Here's how the part is built. I have some questions about the finished solid (model axes, mm). A direction names the side the tool comes from. Round coordinates to 2 decimals unless told otherwise and drop trailing zeros. Order: outer loops, then holes, each group sorted by start corner. A loop starts at its lowest first (then second) coordinate and runs counter-clockwise, first axis right, second up.
```python
from build123d import *

# Parameters (mm, degrees)
F1_W     = 30
F1_H     = 32.3
F2_DEPTH = 7
F0_W     = 12.5
F0_H     = 22.6
F3_DEPTH = 7
F4_W     = 8.75
F4_H     = 4.9
F4_W_2   = 12.5
F4_H_2   = 22.6
F4_H_3   = 4.8
F5_DEPTH = 20


with BuildPart() as f2:
    # F1 (on Top) → F2 (new body)
    with BuildSketch(Plane.XY):
        with Locations((6.25, 11.25)):
            Rectangle(F1_W, F1_H)
    extrude(amount=F2_DEPTH)

    # F0 (on Top) → F3 (cut)
    with BuildSketch(Plane.XY):
        with Locations((6.25, 11.3)):
            Rectangle(F0_W, F0_H)
    extrude(amount=F3_DEPTH, mode=Mode.SUBTRACT)

    # F4 (on Top) → F5 (join)
    with BuildSketch(Plane.XY):
        with Locations((-4.375, -2.45)):
            Rectangle(F4_W, F4_H)
        with Locations((6.25, -2.45)):
            Rectangle(F4_W_2, F4_H)
        with Locations((-4.375, 11.3)):
            Rectangle(F4_W, F4_H_2)
        with Locations((-4.375, 25)):
            Rectangle(F4_W, F4_H_3)
        with Locations((16.875, 11.3)):
            Rectangle(F4_W, F4_H_2)
        with Locations((16.875, -2.45)):
            Rectangle(F4_W, F4_H)
        with Locations((16.875, 25)):
            Rectangle(F4_W, F4_H_3)
    extrude(amount=-F5_DEPTH)


solid = f2.part
```
1) I need wall thicknesses on line 1 (X direction, y = 1, z = -14.5); line 2 (Y direction, x = 6.25, z = -11); line 3 (Z direction, x = 9, y = 26). Which ranges of each line are inside material? Lowest first, please.
2) I'm going to push flat-ended pins straight in: pin 1 (6 mm diameter, centred on x = 8, z = -6, fed in from +Y); pin 2 (5.5 mm diameter, centred on x = 6, y = 25.5, fed in from -Z). Where does each tip first touch, or does it pass through?
3) If we section it at C-C (z = 0.5): Write out the boundary of the cut face in (x, y).
4) If we section it at D-D (z = -3.5): Write out the boundary of the cut face in (x, y), plus the area to 4 significant figures.
5) If we section it at B-B (y = 0.5): Write out the boundary of the cut face in (x, z), plus the area to 4 significant figures.
6) For faces 1 (the flat face through (6, 25, 0)), 2 (the flat face through (13, 11, -20)), 3 (the flat face through (6, 0, -6)), 4 (the flat face through (0, 14, -6)), which set-ups out of +Z, -Z, +X, -X, +Y, -Y let a thin tool reach every point of the face, with its end or its side?
7) If we section it at A-A (x = 3.5): Write out the boundary of the cut face in (y, z).
8) We'd pull the mould along Y, two halves only. Please class faces 5 (the flat face through (6, -4.9, -6)), 6 (the flat face through (-8.75, 11, -6)), 7 (the flat face through (6, 22.6, 3)): +Y half, -Y half, draft (parallel to the pull), parting line (faces both ways), or undercut.
Solutions:
1. line 1: x = -8.75 to 0, 12.5 to 21.25
1. line 2: y = -4.9 to 0
1. line 3: z = 0 to 7
2. pin 1: stops at y = 0
2. pin 2: stops at z = 0
3. outline: (-8.75, -4.9) - (21.25, -4.9) - (21.25, 27.4) - (-8.75, 27.4) - close; hole (0, 0) - (12.5, 0) - (12.5, 22.6) - (0, 22.6) - close
4. outline: (-8.75, -4.9) - (21.25, -4.9) - (21.25, 27.4) - (12.5, 27.4) - (12.5, 0) - (0, 0) - (0, 27.4) - (-8.75, 27.4) - close
4. area: 626.5 mm2
5. outline: (-8.75, -20) - (0, -20) - (0, 7) - (-8.75, 7) - close; (12.5, -20) - (21.25, -20) - (21.25, 7) - (12.5, 7) - close
5. area: 472.5 mm2
6. face 1: -Z, +Y
6. face 2: -Z, +X, -X, +Y, -Y
6. face 3: +Z, -Z
6. face 4: -Z
7. outline: (-4.9, -20) - (0, -20) - (0, 7) - (-4.9, 7) - close; (22.6, 0) - (27.4, 0) - (27.4, 7) - (22.6, 7) - close
8. face 5: -Y half
8. face 6: draft
8. face 7: undercut
